The drawing under review shows one solid part. Ordinate dimensions are in mm from its lowest x, y, z. A direction names the side the tool comes from. Give positions to 0.01 mm unless a question says otherwise; leave off trailing zeros. Loops run counter-clockwise (first coordinate to the right, second up) from the corner with the lowest first, then second, coordinate; pieces in that order, holes last. Notation, with made-up numbers: (72.25, 42) - (119.25, 42) arc R19 ccw to (119.25, 67) - close; hole circle Ø8 at (62, 76). An arc over 180 degrees is marked (long way). Answer as CSV lines item,"result".
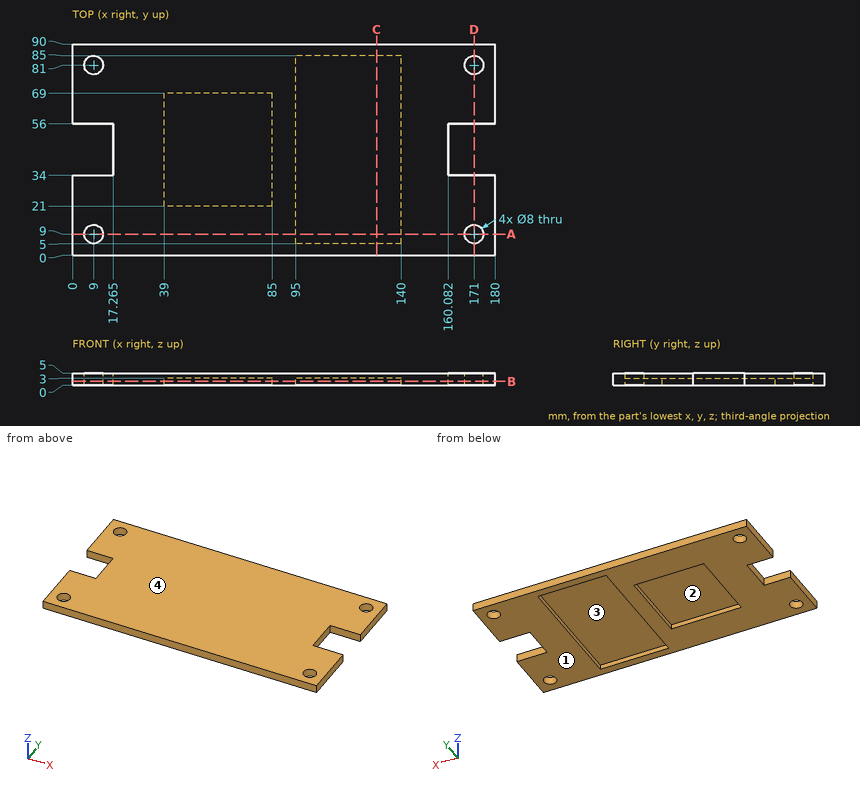
1) Consider section B-B on z = 1.6. Write out the cut boundary in (x, y) (1 decimal).
From the geometry:
outline,"(0, 0) - (180, 0) - (180, 34) - (160.1, 34) - (160.1, 56) - (180, 56) - (180, 90) - (0, 90) - (0, 56) - (17.3, 56) - (17.3, 34) - (0, 34) - close; hole circle Ø8 at (9, 9); hole circle Ø8 at (9, 81); hole (39, 21) - (85, 21) - (85, 69) - (39, 69) - close; hole (95, 5) - (140, 5) - (140, 85) - (95, 85) - close; hole circle Ø8 at (171, 9); hole circle Ø8 at (171, 81)"
2) Machinability: for the marked faces 3 and 4, which of the approach directions +Z, -Z, +X, -X, +Y, -Y give a long, thin tool a straight path to every point of the face, cutting with its end or side? Answer none if there is none.
From the geometry:
face 3,"-Z"
face 4,"+Z, +X, -X, +Y, -Y"
3) Consider section C-C on x = 129.5. Write out the cut boundary in (y, z), and give its area (3 significant figures).
From the geometry:
outline,"(0, 0) - (5, 0) - (5, 3) - (85, 3) - (85, 0) - (90, 0) - (90, 5) - (0, 5) - close"
area,"210 mm^2"
4) Wall thickness on line 1 (X direction, y = 21.5, z = 0.5); line 2 (Y direction, x = 171, z = 3.65); line 3 (X direction, y = 36.5, z = 2.1) (1 decimal): over which ranges is each line inside the solid? List them lowest first. Write a range as from..to.
From the geometry:
line 1,"x = 0..39, 85..95, 140..180"
line 2,"y = 0..5, 13..34, 56..77, 85..90"
line 3,"x = 17.3..39, 85..95, 140..160.1"
5) Consider section D-D on x = 171. Write out the cut boundary in (y, z).
From the geometry:
outline,"(0, 0) - (5, 0) - (5, 5) - (0, 5) - close; (13, 0) - (34, 0) - (34, 5) - (13, 5) - close; (56, 0) - (77, 0) - (77, 5) - (56, 5) - close; (85, 0) - (90, 0) - (90, 5) - (85, 5) - close"
6) Draft analysis for pull direction X (two halves, no side actions). For the marked faces 1 and 2, state which applies: pulls with the +X half, pulls with the -X half, needs draft (parallel to the pull), parting line crosses it, or undercut.
From the geometry:
face 1,"needs draft"
face 2,"undercut"
7) Insertion check: P1, Ø9, axis at x = 171, y = 81, coming from the -Z side; P2, Ø1.5, axis at y = 47.5, z = 1.5, coming from the -X side (1 decimal); P3, Ø2.5, axis at y = 36, z = 1, coming from the +X side; P4, Ø5, axis at x = 171, y = 9, coming from the -Z side. Each pin has a flat end and moves straight along its axis. Give the tip position at first contact, or say it passes through.
From the geometry:
P1,"stops at z = 0"
P2,"stops at x = 17.3"
P3,"stops at x = 160.08"
P4,"passes through"
8) Consider section A-A on y = 9. Write out the cut boundary in (x, z).
From the geometry:
outline,"(0, 0) - (5, 0) - (5, 5) - (0, 5) - close; (13, 0) - (95, 0) - (95, 3) - (140, 3) - (140, 0) - (167, 0) - (167, 5) - (13, 5) - close; (175, 0) - (180, 0) - (180, 5) - (175, 5) - close"
